Geometry: final body of the model. Coordinates: model frame, mm. A direction names the side the tool comes from. Give positions to 0.01 mm unless a question says otherwise; leave off trailing zeros. Write each loop counter-clockwise with the first axis right and the second up, starting at its lowest first coordinate (ties: lowest second). Pieces come first, ordered by that corner, then holes. Notation, with made-up numbers: (-2.75, 34) - (9.25, 34) arc R10 ccw to (9.25, 51) - close; hole circle Ø8 at (54, 43.25). An arc over 180 degrees is marked (long way). Return JSON: item names as keys, results as strings.
from build123d import *

# Parameters (mm, degrees)
BOSS_EXTRUDE1_DEPTH = 12.7
SKETCH3_W           = 5
SKETCH3_H           = 2
CUT_EXTRUDE1_DEPTH  = 75
BOSS_EXTRUDE3_DEPTH = 70


with BuildPart() as part:
    # Sketch1 → Boss-Extrude1 (new body)
    with BuildSketch(Plane(origin=(22.542150286, 0, 0), x_dir=(0, -1, 0), z_dir=(-1, 0, 0))):
        Polygon((-5.910199341, -78.211363822), (8.377300659, -83.411588544), (8.377300659, -86.704627867), (18.219800659, -86.704627867), (18.219800659, 113.295480133), (8.377300659, 113.295480133), (8.377300659, 110.511415536), (-5.910199341, 105.311190814), (-5.910199341, 101.330656125), (8.377300659, 96.130431403), (8.377300659, 90.562302208), (-5.910199341, 85.362077486), (-5.910199341, 81.381542798), (8.377300659, 76.181318076), (8.377300659, 70.613188881), (-5.910199341, 65.412964159), (-5.910199341, 61.43242947), (8.377300659, 56.232204748), (8.377300659, 50.664075553), (-5.910199341, 45.463850831), (-5.910199341, 41.483316143), (8.377300659, 36.283091421), (8.377300659, 30.714962226), (-5.910199341, 25.514737504), (-5.910199341, 21.534202815), (8.377300659, 16.333978093), (8.377300659, 10.765848898), (-5.910199341, 5.565624176), (-5.910199341, 1.585089488), (8.377300659, -3.615135234), (8.377300659, -9.183264429), (-5.910199341, -14.383489151), (-5.910199341, -18.36402384), (8.377300659, -23.564248562), (8.377300659, -29.132377757), (-5.910199341, -34.332602479), (-5.910199341, -38.313137167), (8.377300659, -43.513361889), (8.377300659, -49.081491084), (-5.910199341, -54.281715806), (-5.910199341, -58.262250495), (8.377300659, -63.462475217), (8.377300659, -69.030604412), (-5.910199341, -74.230829134), align=None)
    extrude(amount=-BOSS_EXTRUDE1_DEPTH)

    # Sketch3 → Cut-Extrude1 (cut, symmetric)
    with BuildSketch(Plane.XY):
        with Locations((32.742150286, -12.219800659)):
            Rectangle(SKETCH3_W, SKETCH3_H)
    extrude(amount=CUT_EXTRUDE1_DEPTH, both=True, mode=Mode.SUBTRACT)

    # Sketch4 → Boss-Extrude3 (add)
    with BuildSketch(Plane(origin=(35.242150286, 0, 0), x_dir=(0, 0, -1), z_dir=(1, 0, 0))):
        Polygon((-78, -9.719800659), (-78, -14.719800659), (-68, -14.719800659), (-68, -13.219800659), (-75, -13.219800659), (-75, -11.219800659), (-68, -11.219800659), (-68, -9.719800659), align=None)
        Polygon((68, -14.719800659), (78, -14.719800659), (78, -9.719800659), (68, -9.719800659), (68, -11.219800659), (75, -11.219800659), (75, -13.219800659), (68, -13.219800659), align=None)
    extrude(amount=BOSS_EXTRUDE3_DEPTH)


solid = part.part
Q1. Section query C-C, the plane y = -6. Count the separate pieces of the cut face and the enclosed holes in it, plus the area to 3 significant figures.
Answer key:
{"separate pieces": "10", "enclosed holes": "0", "area": "1,610 mm^2"}
Q2. Pin query (flat end, axial travel): P1, Ø1.6, axis at x = 82.5, y = -12, coming from the +Z side; P2, Ø8, axis at x = 84.5, z = -73.5, coming from the +Y side; P3, Ø1.2, axis at x = 86.5, y = -10.5, coming from the -Z side. Return the tip coordinate at first contact, or that it passes through.
Answer key:
{"P1": "stops at z = 78", "P2": "stops at y = -9.72", "P3": "stops at z = -78"}
Q3. Set-up query: faces 1 (the flat face through (70, -14.72, -73)), 2 (the flat face through (29, -8.377, -6)), 3 (the flat face through (70, -9.72, -73)), 4 (the flat face through (29, -8.377, -85)). Return all of +Z, -Z, +X, -X, +Y, -Y with unobstructed straight access to the full face (end or side cutting, diameter ignored); none if empty.
Answer key:
{"face 1": "+Z, -Z, +X, -Y", "face 2": "+X, -X, +Y", "face 3": "+Z, -Z, +X, +Y", "face 4": "-Z, +X, -X, +Y"}
Q4. Mould query, pull axis Z, two halves, no side actions, for faces 5 (the flat face through (70, -14.72, 73)), 6 (the flat face through (28.803, -1.334, 107.948)), 7 (the flat face through (29, -8.377, 53)), 8 (the flat face through (29, -8.377, 73)). Classes: pulls with the +Z half, pulls with the -Z half, needs draft (parallel to the pull), parting line crosses it, or undercut.
Answer key:
{"face 5": "needs draft", "face 6": "pulls with the +Z half", "face 7": "undercut", "face 8": "undercut"}
Q5. Section query B-B, the plane z = 33.5. Return the cut outline in (x, y).
Answer key:
{"outline": "(22.54, -18.22) - (35.24, -18.22) - (35.24, -13.22) - (30.24, -13.22) - (30.24, -11.22) - (35.24, -11.22) - (35.24, -8.38) - (22.54, -8.38) - close"}
Q6. Material intervals for probe 1 along Z at (x, y) = (89, -11.75); probe 2 along Y at (x, z) = (31, -66.5); probe 3 along Z at (x, y) = (62, -10.75), sorted ascending. Write a range as [from, to].
Answer key:
{"probe 1": "z = [-78, -75], [75, 78]", "probe 2": "y = [-18.22, -13.22], [-11.22, -8.38]", "probe 3": "z = [-78, -68], [68, 78]"}
Q7. Section query A-A, the plane x = 89.5. Return the cut outline in (y, z), plus the area to 3 significant figures.
Answer key:
{"outline": "(-14.72, -78) - (-9.72, -78) - (-9.72, -68) - (-11.22, -68) - (-11.22, -75) - (-13.22, -75) - (-13.22, -68) - (-14.72, -68) - close; (-14.72, 68) - (-13.22, 68) - (-13.22, 75) - (-11.22, 75) - (-11.22, 68) - (-9.72, 68) - (-9.72, 78) - (-14.72, 78) - close", "area": "72.0 mm^2"}
